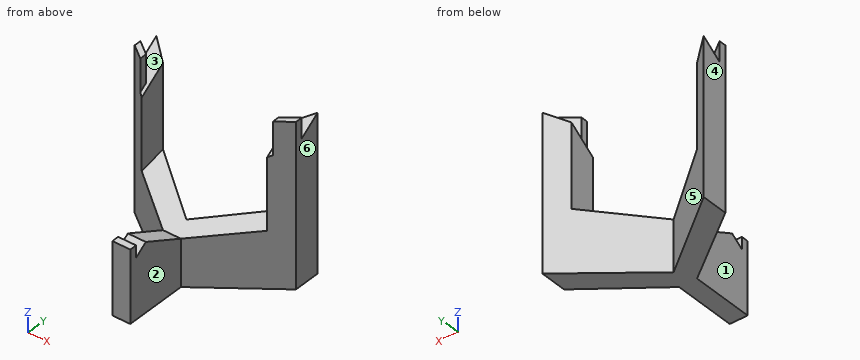
```python
from build123d import *

# Parameters (mm, degrees)
F1_DEPTH      = 80
F3_DEPTH      = 50.001
F3_DEPTH_BACK = 40.001
F5_DEPTH      = 40
F5_DEPTH_BACK = 30
F6_W          = 10
F6_H          = 4
F7_DEPTH      = 30
F9_DEPTH      = 80
F11_DEPTH     = 10


with BuildPart() as f1:
    # F0 (on Top) → F1 (new body)
    with BuildSketch(Plane.XY):
        Polygon((-5, 0), (-5, -35), (5, -35), (5, 0), (45, 30), (45, 45), (0, 10), (-45, 45), (-45, 30), align=None)
    extrude(amount=F1_DEPTH)

    # F2 (on face) → F3 (cut, two sides)
    with BuildSketch(Plane(origin=(-5, 0, 0), x_dir=(0, -1, 0), z_dir=(-1, 0, 0))) as f3_sk:
        Polygon((35, 20.4823592522), (35, 80), (-50, 80), align=None)
    extrude(amount=-F3_DEPTH, mode=Mode.SUBTRACT)
    extrude(f3_sk.sketch, amount=F3_DEPTH_BACK, mode=Mode.SUBTRACT)

    # F4 (on face) → F5 (cut, two sides)
    with BuildSketch(Plane(origin=(-5, 0, 0), x_dir=(0, -1, 0), z_dir=(-1, 0, 0))) as f5_sk:
        Polygon((0, 16), (24.2636963506, 28), (24.2636963506, 88), (-51.7363036494, 88), (-51.7363036494, 28), align=None)
    extrude(amount=-F5_DEPTH, mode=Mode.SUBTRACT)
    extrude(f5_sk.sketch, amount=F5_DEPTH_BACK, mode=Mode.SUBTRACT)

    # F6 (on face) → F7 (join)
    with BuildSketch(Plane(origin=(0, 0, 0), x_dir=(1, 0, 0), z_dir=(0, 0, -1))):
        with Locations((0, 33)):
            Rectangle(F6_W, F6_H)
    extrude(amount=-F7_DEPTH)

    # F8 (on face) → F9 (join)
    with BuildSketch(Plane(origin=(0, 0, 0), x_dir=(1, 0, 0), z_dir=(0, 0, -1))):
        Polygon((-37, -24), (-45, -30), (-45, -34), (-37, -28), align=None)
        Polygon((45, -34), (45, -30), (37, -24), (37, -28), align=None)
    extrude(amount=-F9_DEPTH)

    # F10 (on face) → F11 (join)
    with BuildSketch(Plane(origin=(0, 0, 0), x_dir=(1, 0, 0), z_dir=(0, 0, -1))):
        Polygon((5, 35), (-5, 35), (-5, 0), (-45, -30), (-45, -45), (0, -10), (45, -45), (45, -30), (5, 0), align=None)
    extrude(amount=F11_DEPTH)


solid = f1.part
```
Verification items for the finished model (mm, model axes). Face numbers are marked on the shaded views. A direction names the side the tool comes from. Coordinates: 2 decimals unless noted, no trailing zeros. Loops run counter-clockwise (first coordinate to the right, second up) from the corner with the lowest first, then second, coordinate; pieces in that order, holes last. Notation, with made-up numbers: (-27.75, -38.75) -> (-6.75, -38.75) arc R22 cw to (-6.75, -1.75) -> close; hole circle Ø2 at (81, 48). An arc over 180 degrees is marked (long way). Answer in a Markdown table with one row per item. Add a question column.
1. Section check B-B, the plane y = 15. Enter the section's corners in (x, z), then the cut area to 3 significant figures.
2. Material ranges on probe 1 along X at (y, z) = (32, 2.5); probe 2 along X at (y, z) = (-31, 11); probe 3 along Y at (x, z) = (-30, -2), recorded low to high. Write a range as [from, to].
3. Access from +Z, -Z, +X, -X, +Y, -Y to the whole of each face (thin tool, end or side, straight path). Record for the marked faces 1, 2 and 3.
4. Draft check along X on the marked faces 4, 5 and 6. Enter one of: +X half, -X half, draft (parallel to the pull), parting line (faces both ways), or undercut.
5. Section check D-D, the plane x = -3. Enter the section's corners in (y, z).
6. Section check A-A, the plane z = 57.5. Enter the section's corners in (x, y), then the cut area to 3 significant figures.
7. Section check C-C, the plane z = 6.5. Enter the section's corners in (x, y).
8. Depth check by flat-ended pin: P1, Ø5, axis at y = 27, z = 44, coming from the +X side; P2, Ø3, axis at y = 27, z = 75.5, coming from the +X side; P3, Ø5.5, axis at x = -0.5, z = 25.5, coming from the +Y side. Enter the tip coordinate at first touch or a pass-through.
Derived:
| question | item | result |
|---|---|---|
| 1 | outline | (-25, -10) -> (-6.43, -10) -> (-6.43, 19.48) -> (-25, 19.48) -> close; (6.43, -10) -> (25, -10) -> (25, 19.48) -> (6.43, 19.48) -> close |
| 1 | area | 1,090 mm² |
| 2 | probe 1 | x = [-45, -28.29], [28.29, 45] |
| 2 | probe 2 | x = [-5, 5] |
| 2 | probe 3 | y = [18.75, 33.33] |
| 3 | face 1 | +Z, -Z, -X, -Y |
| 3 | face 2 | +Z, -Z, +X, -Y |
| 3 | face 3 | +Z |
| 4 | face 4 | -X half |
| 4 | face 5 | undercut |
| 4 | face 6 | +X half |
| 5 | outline | (-35, -10) -> (12.33, -10) -> (12.33, 18.86) -> (0, 16) -> (-24.26, 28) -> (-31, 23.28) -> (-31, 30) -> (-35, 30) -> close |
| 6 | outline | (-45, 30) -> (-35, 22.5) -> (-35, 37.22) -> (-45, 45) -> close; (35, 22.5) -> (45, 30) -> (45, 45) -> (35, 37.22) -> close |
| 6 | area | 297 mm² |
| 7 | outline | (-45, 30) -> (-5, 0) -> (-5, -35) -> (5, -35) -> (5, 0) -> (45, 30) -> (45, 45) -> (0, 10) -> (-45, 45) -> close |
| 8 | P1 | stops at x = 44.33 |
| 8 | P2 | stops at x = 43 |
| 8 | P3 | stops at y = -13.65 |
